Source: three-view drawing plus pictorial views. Frame: mm from the lowest corner of the part. A direction names the side the tool comes from. Coordinates: 2 decimals unless noted, no trailing zeros. Order: outer loops, then holes, each group sorted by start corner. A loop starts at its lowest first (then second) coordinate and runs counter-clockwise, first axis right, second up. Notation, with made-up numbers: (44, -32.75) - (82, -32.75) arc R20 cw to (82, -2.75) - close; hole circle Ø9 at (69, 7.5). An arc over 180 degrees is marked (long way). Use a Markdown table: item, result. Add a question column.
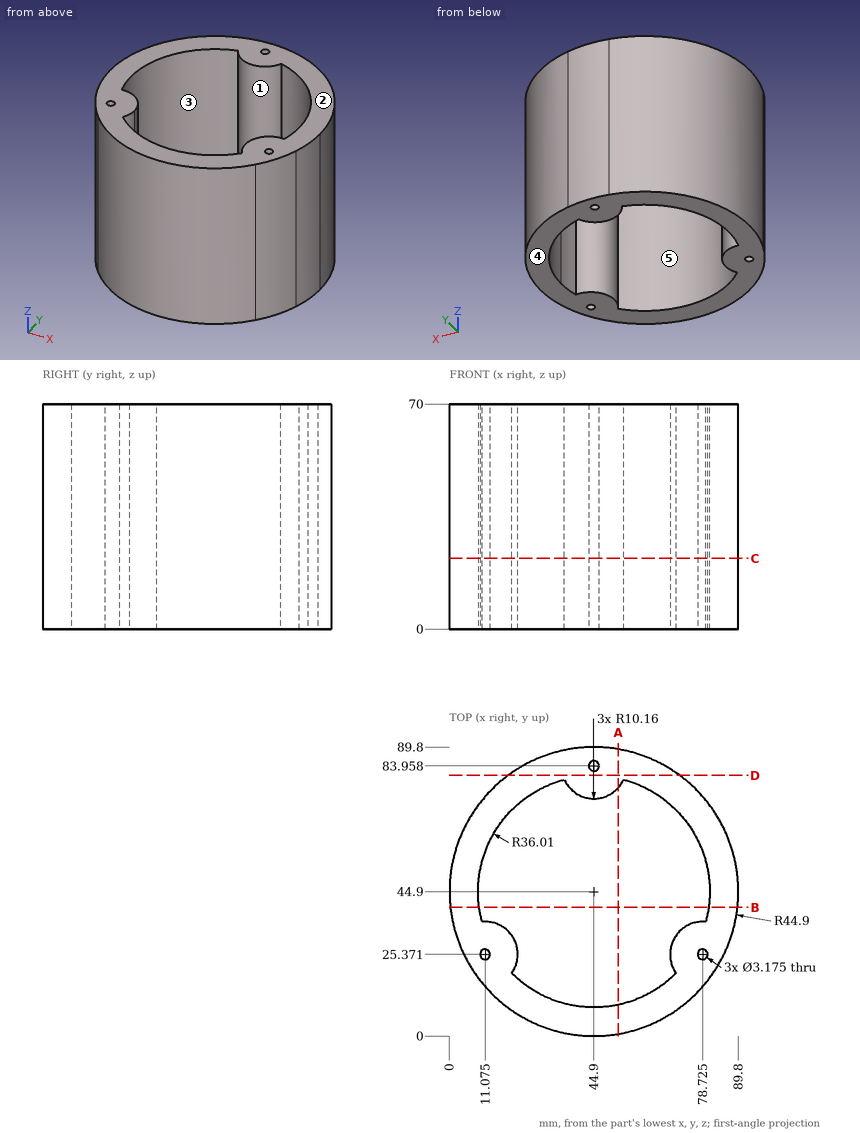
1) Section C-C (z = 22). Return loops of the section in (x, y) (1 decimal).
2) Set-up query: the marked faces 1 and 2. Return all of +Z, -Z, +X, -X, +Y, -Y with unobstructed straight access to the full face (end or side cutting, diameter ignored); none if empty.
3) Section B-B (y = 40). Return loops of the section in (x, z) (1 decimal).
4) Draft query along X for the marked faces 3, 4 and 5. Return one class per face: pulls with the +X half, pulls with the -X half, needs draft (parallel to the pull), parting line crosses it, or undercut.
5) Section A-A (x = 52.5). Return loops of the section in (y, z) (1 decimal).
6) Pin query (flat end, axial travel): pin 1 (12 mm diameter, centred on x = 56.5, z = 55, fed in from +Y); pin 2 (1.5 mm diameter, centred on x = 60.5, z = 18, fed in from +Y); pin 3 (8 mm diameter, centred on x = 53, z = 27.5, fed in from +Y). Return the tip coordinate at first contact, or that it passes through.
7) Section D-D (y = 81). Return loops of the section in (x, z), then the cut area to 3 significant figures.
8) Ray query, line 1 along X through (y, z) = (45, 59.5); line 2 along Y through (x, z) = (20, 16) (1 decimal); line 3 along X through (y, z) = (71, 52.5) (1 decimal). Return the intervals inside material, ascending.
Values follow:
| question | item | result |
|---|---|---|
| 1 | outline | circle Ø89.8 at (44.9, 44.9); hole circle Ø3.2 at (11.1, 25.4); hole (10.1, 35.5) arc R10.2 cw to (19.4, 19.5) arc R36 ccw to (70.4, 19.5) arc R10.2 cw to (79.7, 35.5) arc R36 ccw to (54.1, 79.7) arc R10.2 cw to (35.7, 79.7) arc R36 ccw to start; hole circle Ø3.2 at (44.9, 84); hole circle Ø3.2 at (78.7, 25.4) |
| 2 | face 1 | +Z, -Z |
| 2 | face 2 | +Z, +X, -X, +Y, -Y |
| 3 | outline | (0.3, 0) - (9.2, 0) - (9.2, 70) - (0.3, 70) - close; (80.6, 0) - (89.5, 0) - (89.5, 70) - (80.6, 70) - close |
| 4 | face 3 | undercut |
| 4 | face 4 | needs draft |
| 4 | face 5 | undercut |
| 5 | outline | (0.6, 0) - (9.7, 0) - (9.7, 70) - (0.6, 70) - close; (77.2, 0) - (89.2, 0) - (89.2, 70) - (77.2, 70) - close |
| 6 | pin 1 | stops at y = 89.45 |
| 6 | pin 2 | stops at y = 87.27 |
| 6 | pin 3 | stops at y = 89.61 |
| 7 | outline | (18.2, 0) - (71.6, 0) - (71.6, 70) - (18.2, 70) - close |
| 7 | area | 3,740 mm² |
| 8 | line 1 | x = 0 to 8.89, 80.91 to 89.8 |
| 8 | line 2 | y = 7.5 to 18.9, 20.5 to 30.2, 70.9 to 82.3 |
| 8 | line 3 | x = 8.4 to 20.1, 69.7 to 81.4 |
